Work out the finished part from the listing and answer in its coordinate system (mm). Give positions to 0.01 mm unless a question says otherwise; leave off trailing zeros. Loops run counter-clockwise (first coordinate to the right, second up) from the corner with the lowest first, then second, coordinate; pieces in that order, holes last. Notation, with made-up numbers: (-30, 88.25) - (-7, 88.25) arc R10 cw to (-7, 94.25) - close; hole circle Ø9 at (33, 3). An arc over 180 degrees is marked (long way). One line per item, written item: value.
from build123d import *

# Parameters (mm, degrees)
SKETCH_1_W          = 50
SKETCH_1_H          = 60
EXTRUDE_1_DEPTH     = 2
SKETCH_2_R          = 2.75
SKETCH_2_R_2        = 1.75
CUT_EXTRUDE_1_DEPTH = 3


with BuildPart() as part:
    # 草图1 → 凸台-拉伸1 (new body)
    with BuildSketch(Plane(origin=(0, 0, 0), x_dir=(1, 0, 0), z_dir=(0, 1, 0))):
        with Locations((25, 30)):
            Rectangle(SKETCH_1_W, SKETCH_1_H)
    extrude(amount=EXTRUDE_1_DEPTH)

    # 草图2 → 切除-拉伸1 (cut, through all)
    with BuildSketch(Plane(origin=(0, 2, 0), x_dir=(1, 0, 0), z_dir=(0, 1, 0))):
        with Locations((6, 50)):
            Circle(SKETCH_2_R)
        with Locations((40, 6)):
            Circle(SKETCH_2_R)
        with Locations((12, 15)):
            Circle(SKETCH_2_R_2)
        with Locations((40, 24)):
            Circle(SKETCH_2_R)
        with Locations((22, 50)):
            Circle(SKETCH_2_R)
        Polygon((0, 7.071067812), (7.071067812, 0), (0, 0), align=None)
        Polygon((50, 60), (50, 52.928932188), (42.928932188, 60), align=None)
    extrude(amount=-CUT_EXTRUDE_1_DEPTH, mode=Mode.SUBTRACT)


solid = part.part
1. Find the intervals of material crossed by line 1 along Z through (x, y) = (40, 0.85); line 2 along X through (y, z) = (1.2, -50); line 3 along X through (y, z) = (0.8, -24), in increasing order.
Output:
line 1: z = -60 to -26.75, -21.25 to -8.75, -3.25 to 0
line 2: x = 0 to 3.25, 8.75 to 19.25, 24.75 to 50
line 3: x = 0 to 37.25, 42.75 to 50
2. The mould has two halves that part along X. Classify faces 1 (the cylindrical face through (37.253, 1.014, -6.121)), 2 (the flat face through (25, 0, -30)), 3 (the flat face through (46.514, 1.014, -56.415)): released by +X, released by -X, zero draft, split by the parting line, or undercut.
Output:
face 1: undercut
face 2: zero draft
face 3: released by +X
3. Section B-B (x = 40) is taken. Write down the section's boundary in (y, z).
Output:
outline: (0, -60) - (2, -60) - (2, -26.75) - (0, -26.75) - close; (0, -21.25) - (2, -21.25) - (2, -8.75) - (0, -8.75) - close; (0, -3.25) - (2, -3.25) - (2, 0) - (0, 0) - close
4. Section C-C (z = -24) is taken. Write down the section's boundary in (x, y).
Output:
outline: (0, 0) - (37.25, 0) - (37.25, 2) - (0, 2) - close; (42.75, 0) - (50, 0) - (50, 2) - (42.75, 2) - close
5. Section D-D (x = 22) is taken. Write down the section's boundary in (y, z), and give its area (3 significant figures).
Output:
outline: (0, -60) - (2, -60) - (2, -52.75) - (0, -52.75) - close; (0, -47.25) - (2, -47.25) - (2, 0) - (0, 0) - close
area: 109 mm²
6. Section A-A (y = 1.7) is taken. Write down the section's boundary in (x, z), and give its area (3 significant figures).
Output:
outline: (0, -60) - (42.93, -60) - (50, -52.93) - (50, 0) - (7.07, 0) - (0, -7.07) - close; hole circle Ø5.5 at (6, -50); hole circle Ø3.5 at (12, -15); hole circle Ø5.5 at (22, -50); hole circle Ø5.5 at (40, -24); hole circle Ø5.5 at (40, -6)
area: 2,850 mm²
